Read the model definition and answer for the solid it produces. Units are mm, in the model's axes. Coordinates: 2 decimals unless noted, no trailing zeros. Write each loop counter-clockwise with the first axis right and the second up, starting at its lowest first coordinate (ties: lowest second). Pieces come first, ordered by that corner, then holes. Notation, with made-up numbers: (89, 13) -> (93, 13) arc R15 ccw to (93, 30) -> close; hole circle Ø7 at (59.5, 73). An arc over 180 degrees is marked (long way). Answer as a JSON object with one key per item and string values. Group by question number.
(1) Find section A-A (z = -7). Give the vertices of the cut face in (x, y), then the cut area to 3 significant figures.
(2) Straight lines are drawn through the part: L1, parallel to Z at x = 10.55, y = 0.75; L2, parallel to X at y = 0.6, z = -7.25; L3, parallel to X at y = 1.9, z = -13.5. For each, find the intervals that lie inside material, in ascending order.
(3) Find section C-C (z = -13.25). Give the vertices of the cut face in (x, y), then the cut area to 3 significant figures.
(4) Find section B-B (x = 57.05). Give the vertices of the cut face in (y, z), then the cut area to 3 significant figures.
(5) Flat-ended cylindrical pins translate along their axes: P1, Ø2.5, axis at x = 57.05, z = -7, coming from the -Y side; P2, Ø2.5, axis at x = 10.55, z = -7, coming from the +Y side; P3, Ø0.9, axis at y = 1.5, z = -13.5, coming from the +X side; P4, Ø0.9, axis at x = 1.5, y = 1, coming from the -Z side. Find the tip coordinate at first contact, or state that the pin passes through.
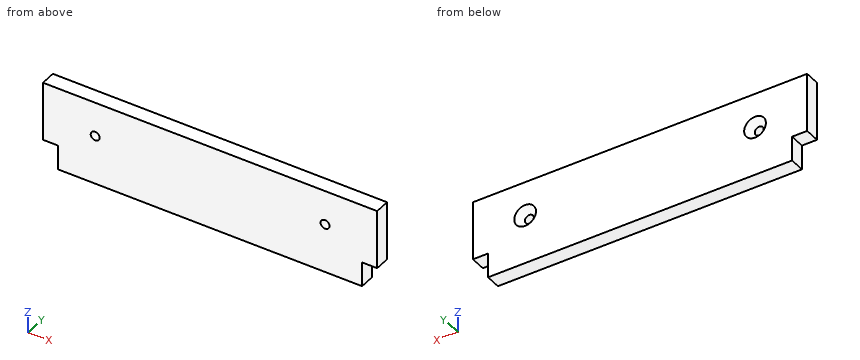
from build123d import *

# Parameters (mm, degrees)
SKETCH1_R                                       = 0.9
BOSS_EXTRUDE1_DEPTH                             = 3.05
CSK_FOR_M2_FLAT_HEAD_MACHINE_SCREW1_D           = 1.8
CSK_FOR_M2_FLAT_HEAD_MACHINE_SCREW1_CSINK_D     = 4.4
CSK_FOR_M2_FLAT_HEAD_MACHINE_SCREW1_CSINK_ANGLE = 90
CSK_FOR_M2_FLAT_HEAD_MACHINE_SCREW2_D           = 1.8
CSK_FOR_M2_FLAT_HEAD_MACHINE_SCREW2_CSINK_D     = 4.4
CSK_FOR_M2_FLAT_HEAD_MACHINE_SCREW2_CSINK_ANGLE = 90


with BuildPart() as part:
    # Sketch1 → Boss-Extrude1 (new body)
    with BuildSketch(Plane(origin=(0, 0, 0), x_dir=(1, 0, 0), z_dir=(0, 1, 0))):
        Polygon((3.05, 17), (3.05, 12), (0, 12), (0, 0), (67.6, 0), (67.6, 12), (64.55, 12), (64.55, 17), align=None)
        with Locations(Location((57.05, 7, 0), (0, 0, 270))):
            Circle(SKETCH1_R, mode=Mode.SUBTRACT)
        with Locations(Location((10.55, 7, 0), (0, 0, 270))):
            Circle(SKETCH1_R, mode=Mode.SUBTRACT)
    extrude(amount=BOSS_EXTRUDE1_DEPTH)

    # CSK for M2 Flat Head Machine Screw1 (through all)
    with Locations(Plane(origin=(0, 3.05, 0), x_dir=(1, 0, 0), z_dir=(0, 1, 0))):
        with Locations((10.55, 7)):
            CounterSinkHole(CSK_FOR_M2_FLAT_HEAD_MACHINE_SCREW1_D / 2, CSK_FOR_M2_FLAT_HEAD_MACHINE_SCREW1_CSINK_D / 2, counter_sink_angle=CSK_FOR_M2_FLAT_HEAD_MACHINE_SCREW1_CSINK_ANGLE)

    # CSK for M2 Flat Head Machine Screw2 (through all)
    with Locations(Plane(origin=(0, 3.05, 0), x_dir=(1, 0, 0), z_dir=(0, 1, 0))):
        with Locations((57.05, 7)):
            CounterSinkHole(CSK_FOR_M2_FLAT_HEAD_MACHINE_SCREW2_D / 2, CSK_FOR_M2_FLAT_HEAD_MACHINE_SCREW2_CSINK_D / 2, counter_sink_angle=CSK_FOR_M2_FLAT_HEAD_MACHINE_SCREW2_CSINK_ANGLE)


solid = part.part
Results below:
{
 "1": {"outline": "(0, 0) -> (9.65, 0) -> (9.65, 1.75) -> (8.35, 3.05) -> (0, 3.05) -> close; (11.45, 0) -> (56.15, 0) -> (56.15, 1.75) -> (54.85, 3.05) -> (12.75, 3.05) -> (11.45, 1.75) -> close; (57.95, 0) -> (67.6, 0) -> (67.6, 3.05) -> (59.25, 3.05) -> (57.95, 1.75) -> close", "area": "192 mm2"},
 "2": {"L1": "z = -17 to -7.9, -6.1 to 0", "L2": "x = 0 to 9.69, 11.41 to 56.19, 57.91 to 67.6", "L3": "x = 3.05 to 64.55"},
 "3": {"outline": "(3.05, 0) -> (64.55, 0) -> (64.55, 3.05) -> (3.05, 3.05) -> close", "area": "188 mm2"},
 "4": {"outline": "(0, -17) -> (3.05, -17) -> (3.05, -9.2) -> (1.75, -7.9) -> (0, -7.9) -> close; (0, -6.1) -> (1.75, -6.1) -> (3.05, -4.8) -> (3.05, 0) -> (0, 0) -> close", "area": "44.7 mm2"},
 "5": {"P1": "stops at y = 0", "P2": "stops at y = 2.1", "P3": "stops at x = 64.55", "P4": "stops at z = -12"}
}
